Build history of the part. All positions in model axes, mm. A direction names the side the tool comes from. Round coordinates to 2 decimals unless told otherwise and drop trailing zeros. Write each loop counter-clockwise with the first axis right and the second up, starting at its lowest first coordinate (ties: lowest second). Pieces come first, ordered by that corner, then holes. Notation, with made-up numbers: M 17.25,25 L 55.25,25 A23 cw 55.25,60 Z; hole C -28,89.5 d3. An arc over 180 degrees is marked long. Write item = value, one per line. Start each with the question number.
Q1. Band-saw the part on C-C on x = -2.1. Write the cut outline in (y, z), plus the area to 3 significant figures.
Q2. Tool access for faces 4 (the cylindrical face through (2.685, -1.13, 0.596)), 5 (the cylindrical face through (-0.45, -6.68, -1.43)): list every direction of +Z, -Z, +X, -X, +Y, -Y with a clear straight run to the whole face (end or side of a thin tool).
Q3. Band-saw the part on B-B on z = 1.9. Write the cut outline in (x, y).
Q4. Probe L1, parallel to X at y = -7, z = 0; L2, parallel to X at y = -7, z = -0.7. List the from-to ranges inside material, lowest first.
Q5. Band-saw the part on A-A on y = -5.75. Write the cut outline in (x, z).
Q6. Pull direction Z, two halves, no side cores. Call faces 1 (the flat face through (1.2, -1.5, -1.2)), 2 (the flat face through (0, -0.8, 0)), 3 (the conical face through (0.397, -13.016, 0.088)): released by +Z, released by -Z, zero draft, split by the parting line, or undercut.
Q7. Drop flat-ended pins along their axis: P1, Ø3, axis at x = -0.5, y = -7, coming from the -Z side; P2, Ø1, axis at y = -4, z = -1.5, coming from the +X side; P3, Ø1, axis at y = -4.5, z = 1, coming from the +X side. Give the stop position or say it passes through.
```python
from build123d import *

# Parameters (mm, degrees)
ENL_V_MAT_EXTRU_1_DEPTH = 0.8


with BuildPart() as part:
    # Esquisse1 → Révolution1 (revolve)
    with BuildSketch(Plane.XY, mode=Mode.PRIVATE) as r_volution1_sk:
        with BuildLine():
            Line((-2.75, -1.5), (-1.5, -1.5))
            Line((-1.5, -1.5), (-1.5, -11.712369611))
            Line((-1.5, -11.712369611), (0, -13.5))
            Line((0, -13.5), (0, 0))
            ThreePointArc((0, 0), (-1.224744871, -0.192113447), (-2.331844763, -0.75))
            Line((-2.331844763, -0.75), (-2.75, -0.75))
            Line((-2.75, -0.75), (-2.75, -1.5))
        make_face()
    revolve(r_volution1_sk.sketch.rotate(Axis((0, -18.848412698, 0), (0, 1, 0)), 270), axis=Axis((0, -18.848412698, 0), (0, 1, 0)))  # turned: the seam where the file's is

    # Esquisse2 → Enlèv. mat.-Extru.1 (cut)
    with BuildSketch(Plane(origin=(0, 0, 0), x_dir=(1, 0, 0), z_dir=(0, 1, 0))):
        Polygon((0, 1.443375673), (-1.25, 0.721687836), (-1.25, -0.721687836), (0, -1.443375673), (1.25, -0.721687836), (1.25, 0.721687836), align=None)
    extrude(amount=-ENL_V_MAT_EXTRU_1_DEPTH, mode=Mode.SUBTRACT)


solid = part.part
```
Conclusion:
q1.outline = M -1.5,-1.78 L -0.75,-1.78 L -0.75,-1.01 A3.4 ccw -0.75,1.01 L -0.75,1.78 L -1.5,1.78 Z
q1.area = 2.87 mm^2
q2.face_4 = +Y, -Y
q2.face_5 = -Y
q3.outline = M -1.99,-1.5 L 1.99,-1.5 L 1.99,-0.75 L 1.35,-0.75 A3.52 ccw -1.35,-0.75 L -1.99,-0.75 Z
q4.L1 = -1.5 to 1.5
q4.L2 = -1.33 to 1.33
q5.outline = C 0,0 d3
q6.face_1 = zero draft
q6.face_2 = undercut
q6.face_3 = split by the parting line
q7.P1 = -1.5
q7.P2 = 1.12
q7.P3 = 1.41
